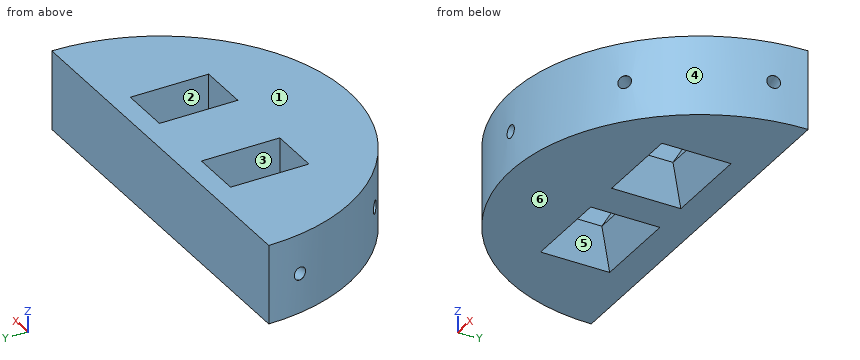
```python
from build123d import *
from OCP.BRepFilletAPI import BRepFilletAPI_MakeChamfer

# Parameters (mm, degrees)
SKETCH1_W           = 16
SKETCH1_H           = 16
BOSS_EXTRUDE1_DEPTH = 25
CIRPATTERN1_COUNT   = 5
CIRPATTERN1_ANGLE   = 160
CHAMFER1_SIZE       = 15
CHAMFER1_SIZE2      = 8.660254038
CHAMFER2_SIZE       = 5.773502692
CHAMFER2_SIZE_2     = 10


with BuildPart() as part:
    # Sketch1 → Boss-Extrude1 (new body)
    with BuildSketch(Plane.XY):
        with BuildLine():
            Line((-119, 0), (0, 0))
            ThreePointArc((0, 0), (-59.5, -59.5), (-119, 0))
        make_face()
        with Locations((-40, -23)):
            Rectangle(SKETCH1_W, SKETCH1_H, mode=Mode.SUBTRACT)
        with Locations((-79, -23)):
            Rectangle(SKETCH1_W, SKETCH1_H, mode=Mode.SUBTRACT)
    extrude(amount=BOSS_EXTRUDE1_DEPTH)

    # Sketch4 → Ø4.0mm Dowel Hole2 (revolve, cut)
    with BuildSketch(Plane(origin=(-0.903938696, -10.332066571, 12.5), x_dir=(0.1736481776669305, 0.9848077530122081, 0), z_dir=(0, 0, 1))):
        Polygon((0, 0), (0, 11.201721238), (2, 10), (2, 0.025), (2.025, 0), align=None)
    f_4_0mm_dowel_hole2 = revolve(axis=Axis((5.349590536, -11.434732499, 12.5), (-0.9848077530122081, 0.1736481776669305, 0)), mode=Mode.SUBTRACT)

    # CirPattern1: Ø4.0mm Dowel Hole2 ×5 about axis
    cirpattern1_axis = Axis((-59.5, 0, 0), (0, 0, -1))
    for i in range(1, CIRPATTERN1_COUNT):
        add(f_4_0mm_dowel_hole2.rotate(cirpattern1_axis, i * CIRPATTERN1_ANGLE / (CIRPATTERN1_COUNT - 1)), mode=Mode.SUBTRACT)

    # Chamfer1: one chamfer whose edges measure the first distance from different faces: ONE call of the kernel's chamfer builder (chamfer() names one face for all edges)
    chamfer1_edges_1 = [part.edges().sort_by_distance(p)[0] for p in [
        (-40, -15, 25),
    ]]
    chamfer1_side_1 = [part.faces().sort_by_distance(p)[0] for p in [
        (-40, -15, 12.5),
    ]]
    chamfer1_edges_2 = [part.edges().sort_by_distance(p)[0] for p in [
        (-79, -15, 25),
    ]]
    chamfer1_side_2 = [part.faces().sort_by_distance(p)[0] for p in [
        (-79, -15, 12.5),
    ]]
    chamfer1 = BRepFilletAPI_MakeChamfer(part.part.solid().wrapped)
    for e in chamfer1_edges_1:
        chamfer1.Add(CHAMFER1_SIZE, CHAMFER1_SIZE2, e.wrapped, chamfer1_side_1[0].wrapped)  # the first distance lies on this face
    for e in chamfer1_edges_2:
        chamfer1.Add(CHAMFER1_SIZE, CHAMFER1_SIZE2, e.wrapped, chamfer1_side_2[0].wrapped)  # the first distance lies on this face
    add(Compound.cast(chamfer1.Shape()), mode=Mode.REPLACE)

    # Chamfer2
    chamfer2_edges_1 = [part.edges().sort_by_distance(p)[0] for p in [
        (-48, -23, 0),
    ]]
    chamfer2_side_1 = [part.faces().sort_by_distance(p)[0] for p in [
        (-48.115470054, -23, 0),
    ]]
    chamfer2_edges_2 = [part.edges().sort_by_distance(p)[0] for p in [
        (-40, -15, 0),
    ]]
    chamfer2_side_2 = [part.faces().sort_by_distance(p)[0] for p in [
        (-40, -14.884529946, 0),
    ]]
    chamfer2_edges_3 = [part.edges().sort_by_distance(p)[0] for p in [
        (-32, -23, 0),
    ]]
    chamfer2_side_3 = [part.faces().sort_by_distance(p)[0] for p in [
        (-31.884529946, -23, 0),
    ]]
    chamfer2_edges_4 = [part.edges().sort_by_distance(p)[0] for p in [
        (-87, -23, 0),
    ]]
    chamfer2_side_4 = [part.faces().sort_by_distance(p)[0] for p in [
        (-87, -23, 0.115470054),
    ]]
    chamfer2_edges_5 = [part.edges().sort_by_distance(p)[0] for p in [
        (-79, -15, 0),
    ]]
    chamfer2_side_5 = [part.faces().sort_by_distance(p)[0] for p in [
        (-79, -14.884529946, 0),
    ]]
    chamfer2_edges_6 = [part.edges().sort_by_distance(p)[0] for p in [
        (-71, -23, 0),
    ]]
    chamfer2_side_6 = [part.faces().sort_by_distance(p)[0] for p in [
        (-70.884529946, -23, 0),
    ]]
    chamfer2 = BRepFilletAPI_MakeChamfer(part.part.solid().wrapped)
    for e in chamfer2_edges_1:
        chamfer2.Add(CHAMFER2_SIZE - 0.0001, CHAMFER2_SIZE_2 - 0.0001, e.wrapped, chamfer2_side_1[0].wrapped)
    for e in chamfer2_edges_2:
        chamfer2.Add(CHAMFER2_SIZE - 0.0001, CHAMFER2_SIZE_2 - 0.0001, e.wrapped, chamfer2_side_2[0].wrapped)
    for e in chamfer2_edges_3:
        chamfer2.Add(CHAMFER2_SIZE - 0.0001, CHAMFER2_SIZE_2 - 0.0001, e.wrapped, chamfer2_side_3[0].wrapped)
    for e in chamfer2_edges_4:
        chamfer2.Add(CHAMFER2_SIZE_2 - 0.0001, CHAMFER2_SIZE - 0.0001, e.wrapped, chamfer2_side_4[0].wrapped)
    for e in chamfer2_edges_5:
        chamfer2.Add(CHAMFER2_SIZE - 0.0001, CHAMFER2_SIZE_2 - 0.0001, e.wrapped, chamfer2_side_5[0].wrapped)
    for e in chamfer2_edges_6:
        chamfer2.Add(CHAMFER2_SIZE - 0.0001, CHAMFER2_SIZE_2 - 0.0001, e.wrapped, chamfer2_side_6[0].wrapped)
    add(Compound.cast(chamfer2.Shape()), mode=Mode.REPLACE)  # a hair under: the kernel refuses the full size


solid = part.part
```
Design review of the part built by this model. Coordinates are the model's own, in mm. Face numbers are marked on the shaded views. A direction names the side the tool comes from. Give positions to 0.01 mm unless a question says otherwise; leave off trailing zeros. Order: outer loops, then holes, each group sorted by start corner. A loop starts at its lowest first (then second) coordinate and runs counter-clockwise, first axis right, second up. Notation, with made-up numbers: (85.5, -39.75) - (130.5, -39.75) arc R24 ccw to (130.5, -26.75) - close; hole circle Ø9 at (-15, 51). An arc over 180 degrees is marked (long way). Use a Markdown table: item, result. Add a question column.
(1) Wall thickness on probe 1 along X at (y, z) = (-39.5, 12.25); probe 2 along Z at (x, y) = (-59.5, -54.5); probe 3 along X at (y, z) = (-27, 7.25): over which ranges is each line inside the solid? List them lowest first. Write a range as [from, to].
(2) Add section D-D on x = -69. Give the boundary of the cut face in (y, z).
(3) Clearance check with flat-ended pins moving along their axes: P1, Ø12, axis at y = -24, z = 14.5, coming from the +X side; P2, Ø12, axis at y = -13.5, z = 14, coming from the +X side; P3, Ø4, axis at x = -77, y = -14, coming from the +Z side. State where each tip first meets the part, or that it passes through.
(4) Mouldability with a two-part tool opening along X and no side actions: class the marked faces 1, 2, 3 and 4 as +X half, -X half, draft (parallel to the pull), parting line (faces both ways), or undercut.
(5) Machinability: for the marked faces 5 and 6, which of the approach directions +Z, -Z, +X, -X, +Y, -Y give a long, thin tool a straight path to every point of the face, cutting with its end or side? Answer none if there is none.
(6) Add section A-A on z = 5. Give the boundary of the cut face in (x, y).
(7) Add section C-C on y = -52. Give the boundary of the cut face in (x, z), then the cut area to 3 significant figures.
Report:
| question | item | result |
|---|---|---|
| 1 | probe 1 | x = [-104, -95.23], [-90.05, -28.95], [-23.77, -15] |
| 1 | probe 2 | z = [0, 10.5], [14.5, 25] |
| 1 | probe 3 | x = [-112.52, -88.59], [-69.41, -49.59], [-30.41, -6.48] |
| 2 | outline | (-58.74, 0) - (-31, 0) - (-31, 6.54) - (-13, 6.54) - (-9.23, 0) - (0, 0) - (0, 25) - (-58.74, 25) - close |
| 3 | P1 | stops at x = -2.79 |
| 3 | P2 | stops at x = -0.47 |
| 3 | P3 | stops at z = 15.2 |
| 4 | face 1 | draft |
| 4 | face 2 | undercut |
| 4 | face 3 | undercut |
| 4 | face 4 | parting line |
| 5 | face 5 | -Z |
| 5 | face 6 | -Z, +X, -X, +Y, -Y |
| 6 | outline | (-119, 0) arc R59.5 ccw to (0, 0) - close; hole (-89.89, -31) - (-68.11, -31) - (-68.11, -12.11) - (-89.89, -12.11) - close; hole (-50.89, -31) - (-29.11, -31) - (-29.11, -12.11) - (-50.89, -12.11) - close |
| 7 | outline | (-88.42, 0) - (-30.58, 0) - (-30.58, 25) - (-88.42, 25) - close; hole circle Ø4 at (-59.5, 12.5) |
| 7 | area | 1,430 mm² |
